```python
from build123d import *

# Parameters (mm, degrees)
BOSS_EXTRUDE1_DEPTH = 42.2
SKETCH2_R           = 1.25
CUT_EXTRUDE1_DEPTH  = 70
FILLET1_R           = 20
BOSS_EXTRUDE2_DEPTH = 2
FILLET2_R           = 10
SKETCH4_R           = 1.25
CUT_EXTRUDE2_DEPTH  = 10


with BuildPart() as part:
    # Sketch1 → Boss-Extrude1 (new body, symmetric)
    with BuildSketch(Plane(origin=(0, 0, 0), x_dir=(0, 0, -1), z_dir=(1, 0, 0))):
        Polygon((0, 0), (0, 82.2), (72, 82.2), (72, 80.2), (2, 80.2), (2, 0), align=None)
    extrude(amount=BOSS_EXTRUDE1_DEPTH, both=True)

    # Sketch2 → Cut-Extrude1 (cut)
    with BuildSketch(Plane.XY):
        with Locations((-30.9, 3.64)):
            Circle(SKETCH2_R)
        with Locations((30.9, 3.64)):
            Circle(SKETCH2_R)
    extrude(amount=-CUT_EXTRUDE1_DEPTH, mode=Mode.SUBTRACT)

    # Fillet1
    fillet1_edges = [part.edges().sort_by_distance(p)[0] for p in [
        (0, 82.2, 0),
        (0, 80.2, -2),
    ]]
    fillet(fillet1_edges, radius=FILLET1_R)

    # Sketch3 → Boss-Extrude2 (add)
    with BuildSketch(Plane.ZY.offset(42.2)):
        with BuildLine():
            Line((-72, 80.2), (-72, 0))
            Line((-72, 0), (-2, 0))
            Line((-2, 0), (-2, 60.2))
            ThreePointArc((-2, 60.2), (-7.857864376, 74.342135624), (-22, 80.2))
            Line((-22, 80.2), (-72, 80.2))
        make_face()
    boss_extrude2 = extrude(amount=-BOSS_EXTRUDE2_DEPTH)

    # Mirror1: Boss-Extrude2 across plane
    add(boss_extrude2.mirror(Plane(origin=(0, 0, 0), x_dir=(0, 0, 1), z_dir=(1, 0, 0))))

    # Fillet2
    fillet2_edges = [part.edges().sort_by_distance(p)[0] for p in [
        (-41.2, 0, -72),
        (41.2, 0, -72),
    ]]
    fillet(fillet2_edges, radius=FILLET2_R)

    # Sketch4 → Cut-Extrude2 (cut)
    with BuildSketch(Plane(origin=(0, 82.2, 0), x_dir=(1, 0, 0), z_dir=(0, 1, 0))):
        with Locations((-30.9, 68.001968)):
            Circle(SKETCH4_R)
        with Locations((30.9, 68.001968)):
            Circle(SKETCH4_R)
    extrude(amount=-CUT_EXTRUDE2_DEPTH, mode=Mode.SUBTRACT)


solid = part.part
```
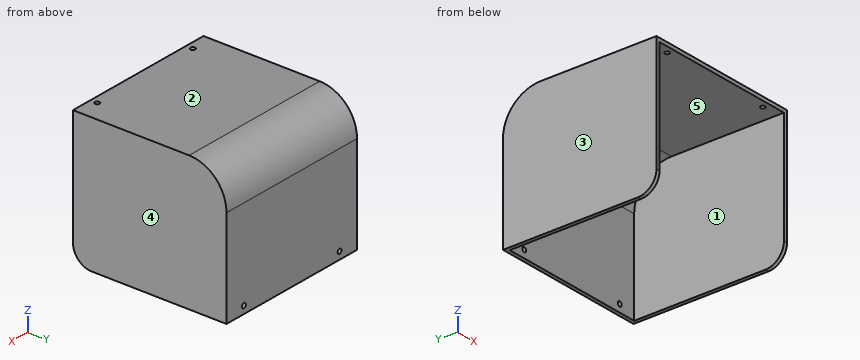
Design review of the part built by this model. Coordinates are the model's own, in mm. Face numbers are marked on the shaded views. A direction names the side the tool comes from. Give positions to 0.01 mm unless a question says otherwise; leave off trailing zeros. Write each loop counter-clockwise with the first axis right and the second up, starting at its lowest first coordinate (ties: lowest second). Pieces come first, ordered by that corner, then holes. Notation, with made-up numbers: (75.25, 29.5) -> (97.25, 29.5) arc R31 cw to (97.25, 53.5) -> close; hole circle Ø2 at (-39, 61.5). An arc over 180 degrees is marked (long way). Answer in a Markdown table with one row per item.
(1) Consider section D-D (y = 51). State the section outline as (x, z) points, then the cut area to 3 significant figures.
Results:
| item | result |
|---|---|
| outline | (-42.2, -72) -> (-40.2, -72) -> (-40.2, -2) -> (40.2, -2) -> (40.2, -72) -> (42.2, -72) -> (42.2, 0) -> (-42.2, 0) -> close |
| area | 449 mm2 |
(2) Mouldability with a two-part tool opening along X and no side actions: class the marked faces 1, 2 and 3 as +X half, -X half, draft (parallel to the pull), parting line (faces both ways), or undercut.
Results:
| item | result |
|---|---|
| face 1 | undercut |
| face 2 | draft |
| face 3 | -X half |
(3) Clearance check with flat-ended pins moving along their axes: pin 1 (12 mm diameter, centred on x = -17.5, y = 65, fed in from +Z); pin 2 (3 mm diameter, centred on x = 24.5, y = 51, fed in from -Z); pin 3 (5 mm diameter, centred on x = -16.5, z = -22.5, fed in from -Y). State where each tip first meets the part, or that it passes through.
Results:
| item | result |
|---|---|
| pin 1 | z = 0 |
| pin 2 | z = -2 |
| pin 3 | y = 80.1 |
(4) For the marked faces 4 and 5, list the 3-axis set-ups (+Z, -Z, +X, -X, +Y, -Y) from which the entire face can be reached by the end or side of a thin tool; tool diameter is ignored.
Results:
| item | result |
|---|---|
| face 4 | +Z, -Z, +X, +Y, -Y |
| face 5 | -Z, -Y |
(5) Consider section B-B (z = -54.5). State the section outline as (x, y) points.
Results:
| item | result |
|---|---|
| outline | (-42.2, 0) -> (-40.2, 0) -> (-40.2, 80.2) -> (40.2, 80.2) -> (40.2, 0) -> (42.2, 0) -> (42.2, 82.2) -> (-42.2, 82.2) -> close |
(6) Consider section C-C (y = 3.64). State the section outline as (x, z) points.
Results:
| item | result |
|---|---|
| outline | (-42.2, -69.72) -> (-40.2, -69.72) -> (-40.2, -2) -> (-32.15, -2) -> (-32.15, 0) -> (-42.2, 0) -> close; (-29.65, -2) -> (29.65, -2) -> (29.65, 0) -> (-29.65, 0) -> close; (32.15, -2) -> (40.2, -2) -> (40.2, -69.72) -> (42.2, -69.72) -> (42.2, 0) -> (32.15, 0) -> close |
(7) To check wall thickness, follow probe 1 along X at (y, z) = (61, -58); probe 2 along Y at (x, z) = (18, -54); probe 3 along Z at (x, y) = (31, 24). State the ranges of each line that lie inside material, in increasing order.
Results:
| item | result |
|---|---|
| probe 1 | -42.2 to -40.2, 40.2 to 42.2 |
| probe 2 | 80.2 to 82.2 |
| probe 3 | -2 to 0 |
(8) Consider section A-A (x = 30.9). State the section outline as (y, z) points.
Results:
| item | result |
|---|---|
| outline | (0, -2) -> (2.39, -2) -> (2.39, 0) -> (0, 0) -> close; (4.89, -2) -> (60.2, -2) arc R20 cw to (80.2, -22) -> (80.2, -66.75) -> (82.2, -66.75) -> (82.2, -20) arc R20 ccw to (62.2, 0) -> (4.89, 0) -> close; (80.2, -72) -> (82.2, -72) -> (82.2, -69.25) -> (80.2, -69.25) -> close |
